CAD build for the part. Positions are in the model's coordinates, mm. Face numbers are marked on the shaded views. A direction names the side the tool comes from. Round coordinates to 2 decimals unless told otherwise and drop trailing zeros. Order: outer loops, then holes, each group sorted by start corner. A loop starts at its lowest first (then second) coordinate and runs counter-clockwise, first axis right, second up. Notation, with made-up numbers: (85.25, 79) - (96.25, 79) arc R18 ccw to (96.25, 90) - close; hole circle Ø11 at (4, 16.5). An arc over 180 degrees is marked (long way). Use one line per item in the form item = value. Start each with the question number.
from build123d import *

# Parameters (mm, degrees)
SKETCH_1_W          = 25
SKETCH_1_H          = 22
SKETCH_1_R          = 7.5
EXTRUDE_1_DEPTH     = 25
SKETCH_2_W          = 20
SKETCH_2_H          = 3
EXTRUDE_2_DEPTH     = 25
SKETCH_3_R          = 3.15
CUT_EXTRUDE_1_DEPTH = 25
FILLET_2_R          = 10
SKETCH_4_W          = 6
SKETCH_4_H          = 6
CUT_EXTRUDE_2_DEPTH = 25
FILLET_3_R          = 10
FILLET_4_R          = 10
SKETCH_5_W          = 21.715962642
SKETCH_5_H          = 3
CUT_EXTRUDE_3_DEPTH = 25
FILLET_5_R          = 4
SKETCH_8_W          = 25
SKETCH_8_H          = 3.5
EXTRUDE_3_DEPTH     = 3
SKETCH_6_R          = 2.15
CUT_EXTRUDE_4_DEPTH = 25
CHAMFER_1_SIZE      = 6


with BuildPart() as part:
    # 草图1 → 凸台-拉伸1 (new body)
    with BuildSketch(Plane.XY):
        Rectangle(SKETCH_1_W, SKETCH_1_H)
        with Locations((2.5, 0)):
            Circle(SKETCH_1_R, mode=Mode.SUBTRACT)
    extrude(amount=EXTRUDE_1_DEPTH)

    # 草图2 → 凸台-拉伸2 (add)
    with BuildSketch(Plane(origin=(12.5, 0, 0), x_dir=(0, 0, -1), z_dir=(1, 0, 0))):
        with Locations((-15, 3.65)):
            Rectangle(SKETCH_2_W, SKETCH_2_H)
        with Locations((-15, -3.65)):
            Rectangle(SKETCH_2_W, SKETCH_2_H)
    extrude(amount=EXTRUDE_2_DEPTH)

    # 草图3 → 切除-拉伸1 (cut)
    with BuildSketch(Plane(origin=(0, 5.15, 0), x_dir=(1, 0, 0), z_dir=(0, 1, 0))):
        with Locations(Location((29.5, -15, 0), (0, 0, 270))):
            Circle(SKETCH_3_R)
    extrude(amount=-CUT_EXTRUDE_1_DEPTH, mode=Mode.SUBTRACT)

    # 圆角2
    # the kernel refuses this fillet: 10 mm, written as the material it adds along each edge
    with BuildSketch(Plane(origin=(12.5, 5.15, 5), x_dir=(0, 0, -1), z_dir=(0, -1, 0)), Plane(origin=(12.5, -2.15, 5), x_dir=(0, 0, -1), z_dir=(0, -1, 0))) as fillet_2_piece_1:
        with BuildLine():
            CenterArc((10, 8.660254038), FILLET_2_R, 180, 60)
            Line((0, 8.660254038), (-0.2, 8.660254038))
            Line((-0.2, 8.660254038), (-0.2, 0))
            Line((-0.2, 0), (0, -0.2))
            ThreePointArc((0, -0.2), (2.5, -0.2), (4.9, -0.173205081))
            Line((4.9, -0.173205081), (5, 0))
        make_face()
    extrude(amount=3)
    with BuildSketch(Plane(origin=(12.5, 5.15, 5), x_dir=(0, 0, -1), z_dir=(0, -1, 0))) as fillet_2_piece_2_section:
        with BuildLine():
            CenterArc((10, 8.660254038), FILLET_2_R, 180, 60)
            Line((0, 8.660254038), (-0.2, 8.660254038))
            Line((-0.2, 8.660254038), (-0.2, 0))
            Line((-0.2, 0), (0, -0.2))
            ThreePointArc((0, -0.2), (2.5, -0.2), (4.9, -0.173205081))
            Line((4.9, -0.173205081), (5, 0))
        make_face()
    fillet_2_piece_2 = extrude(amount=24.650635095, mode=Mode.PRIVATE)
    fillet_2_piece_2 = split(fillet_2_piece_2, bisect_by=Plane(origin=(14.663104458, -5.15, 3.704832889), z_dir=(0, 1, 0)), keep=Keep.TOP, mode=Mode.PRIVATE)
    fillet_2_piece_2 = split(fillet_2_piece_2, bisect_by=Plane(origin=(14.663104458, -2.15, 3.704832889), z_dir=(0, -1, 0)), keep=Keep.TOP, mode=Mode.PRIVATE)
    add(fillet_2_piece_2)
    with BuildSketch(Plane(origin=(12.5, 19.500635095, 5), x_dir=(0, 0, -1), z_dir=(0, -1, 0))) as fillet_2_piece_3_section:
        with BuildLine():
            CenterArc((10, 8.660254038), FILLET_2_R, 180, 60)
            Line((0, 8.660254038), (-0.2, 8.660254038))
            Line((-0.2, 8.660254038), (-0.2, 0))
            Line((-0.2, 0), (0, -0.2))
            ThreePointArc((0, -0.2), (2.5, -0.2), (4.9, -0.173205081))
            Line((4.9, -0.173205081), (5, 0))
        make_face()
    fillet_2_piece_3 = extrude(amount=24.650635095, mode=Mode.PRIVATE)
    fillet_2_piece_3 = split(fillet_2_piece_3, bisect_by=Plane(origin=(14.663104458, 2.15, 3.704832889), z_dir=(0, 1, 0)), keep=Keep.TOP, mode=Mode.PRIVATE)
    fillet_2_piece_3 = split(fillet_2_piece_3, bisect_by=Plane(origin=(14.663104458, 5.15, 3.704832889), z_dir=(0, -1, 0)), keep=Keep.TOP, mode=Mode.PRIVATE)
    add(fillet_2_piece_3)

    # 草图4 → 切除-拉伸2 (cut)
    with BuildSketch(Plane(origin=(0, 0, 0), x_dir=(-1, 0, 0), z_dir=(0, 0, -1))):
        with Locations((9.5, 8)):
            Rectangle(SKETCH_4_W, SKETCH_4_H)
        with Locations((9.5, -8)):
            Rectangle(SKETCH_4_W, SKETCH_4_H)
    extrude(amount=-CUT_EXTRUDE_2_DEPTH, mode=Mode.SUBTRACT)

    # 圆角3
    # the kernel refuses this fillet: 10 mm, written as the material it takes off along each edge
    with BuildSketch(Plane(origin=(-6.5, -11, -22.912878475), x_dir=(0, 1, 0), z_dir=(0, 0, 1))) as fillet_3_piece_1:
        with BuildLine():
            CenterArc((10, -9.16515139), FILLET_3_R, 113.578178478, 66.421821522)
            Line((0, -9.16515139), (-0.2, -9.16515139))
            Line((-0.2, -9.16515139), (-0.2, 0))
            Line((-0.2, 0), (0, 0.2))
            ThreePointArc((0, 0.2), (3, 0.2), (5.92, 0.183303028))
            Line((5.92, 0.183303028), (6, 0))
        make_face()
    extrude(amount=70.82575695, mode=Mode.SUBTRACT)
    with BuildSketch(Plane(origin=(-6.5, 11, -22.912878475), x_dir=(1, 0, 0), z_dir=(0, 0, 1))) as fillet_3_piece_2:
        with BuildLine():
            CenterArc((9.16515139, -10), FILLET_3_R, 90, 66.421821522)
            Line((0, -6), (-0.183303028, -5.92))
            ThreePointArc((-0.183303028, -5.92), (-0.2, -3), (-0.2, 0))
            Line((-0.2, 0), (0, 0.2))
            Line((0, 0.2), (9.16515139, 0.2))
            Line((9.16515139, 0.2), (9.16515139, 0))
        make_face()
    extrude(amount=70.82575695, mode=Mode.SUBTRACT)

    # 圆角4
    # the kernel refuses this fillet: 10 mm, written as the material it takes off along each edge
    with BuildSketch(Plane(origin=(12.5, 11, -22.745535276), x_dir=(0, -1, 0), z_dir=(0, 0, 1))) as fillet_4_piece_1:
        with BuildLine():
            CenterArc((10, -9.09821411), FILLET_4_R, 114.519316483, 65.480683517)
            Line((0, -9.09821411), (-0.2, -9.09821411))
            Line((-0.2, -9.09821411), (-0.2, 0))
            Line((-0.2, 0), (0, 0.2))
            ThreePointArc((0, 0.2), (2.925, 0.2), (5.767, 0.181964282))
            Line((5.767, 0.181964282), (5.85, 0))
        make_face()
    extrude(amount=70.491070552, mode=Mode.SUBTRACT)
    with BuildSketch(Plane(origin=(12.5, -11, -22.745535276), x_dir=(-1, 0, 0), z_dir=(0, 0, 1))) as fillet_4_piece_2:
        with BuildLine():
            CenterArc((9.09821411, -10), FILLET_4_R, 90, 65.480683517)
            Line((0, -5.85), (-0.181964282, -5.767))
            ThreePointArc((-0.181964282, -5.767), (-0.2, -2.925), (-0.2, 0))
            Line((-0.2, 0), (0, 0.2))
            Line((0, 0.2), (9.09821411, 0.2))
            Line((9.09821411, 0.2), (9.09821411, 0))
        make_face()
    extrude(amount=70.491070552, mode=Mode.SUBTRACT)

    # 草图5 → 切除-拉伸3 (cut)
    with BuildSketch(Plane(origin=(0, 0, 0), x_dir=(-1, 0, 0), z_dir=(0, 0, -1))):
        with Locations((12.5, 0)):
            Rectangle(SKETCH_5_W, SKETCH_5_H)
    extrude(amount=-CUT_EXTRUDE_3_DEPTH, mode=Mode.SUBTRACT)

    # 圆角5
    fillet_5_edges = [part.edges().sort_by_distance(p)[0] for p in [
        (-4.848469228, -1.5, 12.5),
        (-4.848469228, 1.5, 12.5),
    ]]
    fillet(fillet_5_edges, radius=FILLET_5_R)

    # 草图8 → 凸台-拉伸3 (add)
    with BuildSketch(Plane.ZY.offset(12.5)):
        with Locations((12.5, 3.25)):
            Rectangle(SKETCH_8_W, SKETCH_8_H)
        with Locations((12.5, -3.25)):
            Rectangle(SKETCH_8_W, SKETCH_8_H)
    extrude(amount=EXTRUDE_3_DEPTH)

    # 草图6 → 切除-拉伸4 (cut)
    with BuildSketch(Plane(origin=(0, 5, 0), x_dir=(1, 0, 0), z_dir=(0, 1, 0))):
        with Locations(Location((-11, -7, 0), (0, 0, 180))):
            Circle(SKETCH_6_R)
        with Locations(Location((-11, -18, 0), (0, 0, 180))):
            Circle(SKETCH_6_R)
    extrude(amount=-CUT_EXTRUDE_4_DEPTH, mode=Mode.SUBTRACT)

    # 倒角1
    chamfer_1_edges = [part.edges().sort_by_distance(p)[0] for p in [
        (37.5, 3.65, 25),
        (37.5, 3.65, 5),
        (37.5, -3.65, 25),
        (37.5, -3.65, 5),
    ]]
    chamfer(chamfer_1_edges, length=CHAMFER_1_SIZE)


solid = part.part
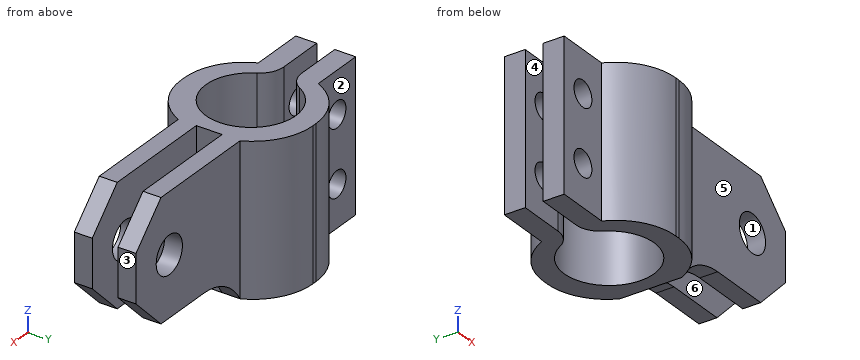
(1) Wall check: line 1 (Z direction, x = -11, y = -2.15); line 2 (Y direction, x = 2.5, z = 8.75); line 3 (Y direction, x = -8, z = 14). Give the ranges that are in metal, low to high. Write a range as [from, to].
(2) Mould opens along X. For the marked faces 1, 2 and 3 say: pulls with the +X half, pulls with the -X half, needs draft (parallel to the pull), parting line crosses it, or undercut.
(3) Which spindle directions (+Z, -Z, +X, -X, +Y, -Y) get a long thin tool onto all of the face, cutting with end or side? Do the marked faces 4, 5 and 6. Say none if no direction does.
(4) Slice it at B-B (z = 15). Give the number of separate pieces and of enclosed holes in the cut face, and give its area (3 significant figures).
(5) Flat gauge pins, fed straight in: P1, Ø5, axis at x = 29.5, z = 15, coming from the +Y side; P2, Ø2, axis at y = 1, z = 9.5, coming from the +X side; P3, Ø3.5, axis at x = 25, y = -3.5, coming from the -Z side; P4, Ø6.5, axis at x = -13, z = 9, coming from the -Y side. Where does each tip first touch, or does it go through?
(6) Slice it at A-A (x = -11). Give the cut face in (y, z), and give its area (3 significant figures).
(7) Slice it at D-D (x = 9). Give the cut face in (y, z).
(8) Slice it at C-C (x = 29.5). Give the cut face in (y, z).
Results list:
q1.line_1 = [0, 4.85], [9.15, 15.85], [20.15, 25]
q1.line_2 = [-11, -7.5], [7.5, 11]
q1.line_3 = [-5, -1.5], [1.5, 5]
q2.face_1 = undercut
q2.face_2 = needs draft
q2.face_3 = pulls with the +X half
q3.face_4 = +Z, -Z, -X
q3.face_5 = +Z, -Z, +X, -Y
q3.face_6 = +Z, -Z, +X
q4.separate_pieces = 3
q4.enclosed_holes = 0
q4.area = 349 mm²
q5.P1 = through
q5.P2 = 12.5
q5.P3 = 5
q5.P4 = -5
q6.outline = (-5, 0) - (-1.5, 0) - (-1.5, 4.85) - (-5, 4.85) - close; (-5, 9.15) - (-1.5, 9.15) - (-1.5, 15.85) - (-5, 15.85) - close; (-5, 20.15) - (-1.5, 20.15) - (-1.5, 25) - (-5, 25) - close; (1.5, 0) - (5, 0) - (5, 4.85) - (1.5, 4.85) - close; (1.5, 9.15) - (5, 9.15) - (5, 15.85) - (1.5, 15.85) - close; (1.5, 20.15) - (5, 20.15) - (5, 25) - (1.5, 25) - close
q6.area = 115 mm²
q7.outline = (-9.29, 0) - (-3.74, 0) - (-3.74, 25) - (-9.29, 25) - close; (3.74, 0) - (9.29, 0) - (9.29, 25) - (3.74, 25) - close
q8.outline = (-5.15, 5) - (-2.15, 5) - (-2.15, 11.85) - (-5.15, 11.85) - close; (-5.15, 18.15) - (-2.15, 18.15) - (-2.15, 25) - (-5.15, 25) - close; (2.15, 5) - (5.15, 5) - (5.15, 11.85) - (2.15, 11.85) - close; (2.15, 18.15) - (5.15, 18.15) - (5.15, 25) - (2.15, 25) - close
